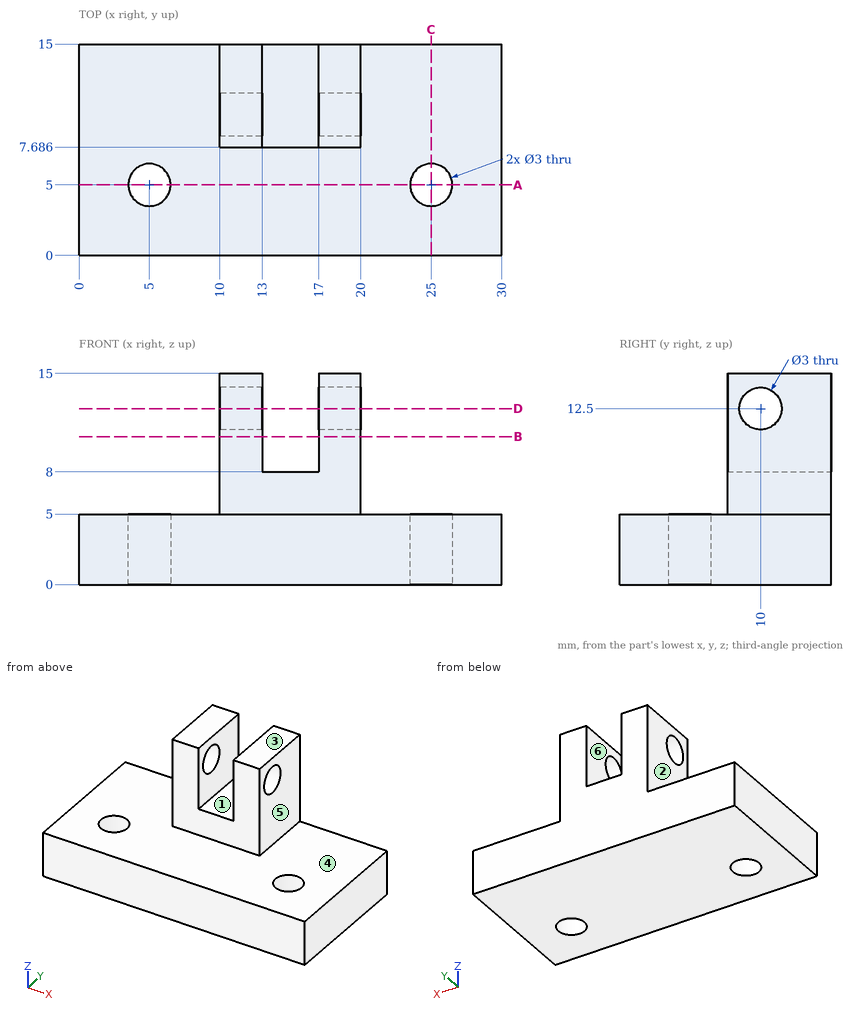
The drawing under review shows one solid part. Ordinate dimensions are in mm from its lowest x, y, z. A direction names the side the tool comes from. Round coordinates to 2 decimals unless told otherwise and drop trailing zeros. Loops run counter-clockwise (first coordinate to the right, second up) from the corner with the lowest first, then second, coordinate; pieces in that order, holes last. Notation, with made-up numbers: (67.5, 24) - (120.5, 24) arc R24 ccw to (120.5, 50) - close; hole circle Ø4 at (69, 38). An arc over 180 degrees is marked (long way). One line per item, written item: value. Start each with the question number.
1) Consider section A-A on y = 5. Give the boundary of the cut face in (x, z).
2) Consider section D-D on z = 12.5. Give the boundary of the cut face in (x, y), then the cut area to 3 significant figures.
3) Consider section B-B on z = 10.5. Give the boundary of the cut face in (x, y), then the cut area to 3 significant figures.
4) To check wall thickness, follow L1, parallel to Z at x = 11.25, y = 10; L2, parallel to X at y = 12.5, z = 8.5; L3, parallel to Z at x = 13.5, y = 12.75. State the ranges of each line that lie inside material, in increasing order. Write a range as from..to.
5) Consider section C-C on x = 25. Give the boundary of the cut face in (y, z), then the cut area to 3 significant figures.
6) Insertion check: pin 1 Ø7.5 at (y, z) = (10.5, 13) entering from -X; pin 2 Ø2.5 at (x, y) = (25, 5) entering from +Z; pin 3 Ø2 at (y, z) = (13, 11) entering from +X; pin 4 Ø1.5 at (x, z) = (17.5, 8.5) entering from -Y. Each pin has a flat end and moves straight along its axis. Give the tip position at first contact, or say it passes through.
7) For the marked faces 4, 5 and 6, list the 3-axis set-ups (+Z, -Z, +X, -X, +Y, -Y) from which the entire face can be reached by the end or side of a thin tool; tool diameter is ignored.
8) Draft analysis for pull direction X (two halves, no side actions). For the marked faces 1, 2 and 3, state which applies: +X half, -X half, draft (parallel to the pull), parting line (faces both ways), or undercut.
Reported:
1. outline: (0, 0) - (3.5, 0) - (3.5, 5) - (0, 5) - close; (6.5, 0) - (23.5, 0) - (23.5, 5) - (6.5, 5) - close; (26.5, 0) - (30, 0) - (30, 5) - (26.5, 5) - close
2. outline: (10, 7.69) - (13, 7.69) - (13, 8.5) - (10, 8.5) - close; (10, 11.5) - (13, 11.5) - (13, 15) - (10, 15) - close; (17, 7.69) - (20, 7.69) - (20, 8.5) - (17, 8.5) - close; (17, 11.5) - (20, 11.5) - (20, 15) - (17, 15) - close
2. area: 25.9 mm^2
3. outline: (10, 7.69) - (13, 7.69) - (13, 15) - (10, 15) - close; (17, 7.69) - (20, 7.69) - (20, 15) - (17, 15) - close
3. area: 43.9 mm^2
4. L1: z = 0..11, 14..15
4. L2: x = 10..13, 17..20
4. L3: z = 0..8
5. outline: (0, 0) - (3.5, 0) - (3.5, 5) - (0, 5) - close; (6.5, 0) - (15, 0) - (15, 5) - (6.5, 5) - close
5. area: 60.0 mm^2
6. pin 1: stops at x = 10
6. pin 2: passes through
6. pin 3: stops at x = 20
6. pin 4: stops at y = 7.69
7. face 4: +Z, -Y
7. face 5: +Z, +X, +Y, -Y
7. face 6: +Z, +Y, -Y
8. face 1: undercut
8. face 2: -X half
8. face 3: draft
